Geometry check sheet. Reference: the model listing, model coordinates, mm. A direction names the side the tool comes from. Round coordinates to 2 decimals unless told otherwise and drop trailing zeros. Loops run counter-clockwise (first coordinate to the right, second up) from the corner with the lowest first, then second, coordinate; pieces in that order, holes last. Notation, with made-up numbers: (34, 25.25) -> (93, 25.25) arc R16 ccw to (93, 42.25) -> close; hole circle Ø6 at (16, -28). An arc over 180 degrees is marked (long way). Use a Markdown table: item, result. Add a question column.
Q1. Gauge pin test, flat ends, axial feed: P1, Ø3, axis at x = -22, z = 60, coming from the -Y side; P2, Ø12, axis at x = 9.5, z = 20, coming from the -Y side; P3, Ø5, axis at x = 15.5, y = -46.5, coming from the +Z side. Record the tip position at first contact, or that the pin passes through.
Q2. Material ranges on L1, parallel to Y at x = 0, z = 2.95; L2, parallel to Z at x = 40, y = -7; L3, parallel to Y at x = 0.5, z = 25, recorded low to high.
Q3. Sectioned sample at D-D, the plane x = 25.5. Enter the section's corners in (y, z).
Q4. Sectioned sample at A-A, the plane y = 0. Enter the section's corners in (x, z).
Q5. Set-up check for faces 1 (the face through (21.44, 6.75, 46.37)), 2 (the face through (0, 0, 91.44)): record each of +Z, -Z, +X, -X, +Y, -Y from which the full face is reachable in a straight line by a thin tool's end or side.
Q6. Sectioned sample at C-C, the plane z = 11.5. Enter the section's corners in (x, y).
Q7. Release check for a two-part mould opening along X. For faces 3 (the face through (55.3, 17.41, 3.17)), 4 (the face through (-13.119, -59.077, 1.878)), 5 (the face through (-1, -25, 2.54)), 6 (the face through (4, -58, 3.81)) record: released by +X, released by -X, zero draft, split by the parting line, or undercut.
```python
from build123d import *

# Parameters (mm, degrees)
F0_R     = 60.516336
F1_DEPTH = 3.81
F2_T     = -2.54
F3_R     = 22.478017
F4_DEPTH = 88.9


with BuildPart() as f1:
    # F0 (on Top) → F1 (new body)
    with BuildSketch(Plane.XY):
        Circle(F0_R)
    extrude(amount=F1_DEPTH)

    # F2
    f2_openings = [f1.faces().sort_by_distance(p)[0] for p in [
        (0, 0, 3.81),
    ]]
    offset(amount=F2_T, openings=f2_openings)

    # F3 (on face) → F4 (join)
    with BuildSketch(Plane.XY.offset(2.54)):
        Circle(F3_R)
    extrude(amount=F4_DEPTH)


solid = f1.part
```
Values:
| question | item | result |
|---|---|---|
| 1 | P1 | y = -9.22 |
| 1 | P2 | y = -22.2 |
| 1 | P3 | z = 2.54 |
| 2 | L1 | -60.52 to -57.98, -22.48 to 22.48, 57.98 to 60.52 |
| 2 | L2 | 0 to 2.54 |
| 2 | L3 | -22.47 to 22.47 |
| 3 | outline | (-54.88, 0) -> (54.88, 0) -> (54.88, 3.81) -> (52.07, 3.81) -> (52.07, 2.54) -> (-52.07, 2.54) -> (-52.07, 3.81) -> (-54.88, 3.81) -> close |
| 4 | outline | (-60.52, 0) -> (60.52, 0) -> (60.52, 3.81) -> (57.98, 3.81) -> (57.98, 2.54) -> (22.48, 2.54) -> (22.48, 91.44) -> (-22.48, 91.44) -> (-22.48, 2.54) -> (-57.98, 2.54) -> (-57.98, 3.81) -> (-60.52, 3.81) -> close |
| 5 | face 1 | +Z |
| 5 | face 2 | +Z, +X, -X, +Y, -Y |
| 6 | outline | circle Ø44.96 at (0, 0) |
| 7 | face 3 | undercut |
| 7 | face 4 | split by the parting line |
| 7 | face 5 | undercut |
| 7 | face 6 | zero draft |
